The listing builds one solid part. Answer for the finished solid, in the listing's coordinates (mm). A direction names the side the tool comes from. Round coordinates to 2 decimals unless told otherwise and drop trailing zeros. Loops run counter-clockwise (first coordinate to the right, second up) from the corner with the lowest first, then second, coordinate; pieces in that order, holes last. Notation, with made-up numbers: M 22.5,27.25 L 70.5,27.25 A22 ccw 70.5,64.25 Z; hole C 75.25,81 d11. An arc over 180 degrees is marked long. Answer as a JSON object with one key per item and string values.
```python
from build123d import *

# Parameters (mm, degrees)
SKETCH1_R           = 48.26
BOSS_EXTRUDE1_DEPTH = 25.4
SKETCH2_R           = 8.382
CUT_EXTRUDE1_DEPTH  = 5.334
SKETCH12_R          = 6.731
CUT_EXTRUDE5_DEPTH  = 73.823177629
SKETCH15_R          = 6.731
BOSS_EXTRUDE2_DEPTH = 5.08
SKETCH16_R          = 1.5
CUT_EXTRUDE9_DEPTH  = 75.746809965
SKETCH14_R          = 6.858
CUT_EXTRUDE8_DEPTH  = 73.823177629


with BuildPart() as part:
    # Sketch1 → Boss-Extrude1 (new body)
    with BuildSketch(Plane.XY):
        Circle(SKETCH1_R)
    extrude(amount=BOSS_EXTRUDE1_DEPTH)

    # Sketch2 → Cut-Extrude1 (cut)
    with BuildSketch(Plane.XY.offset(25.4)):
        Circle(SKETCH2_R)
    cut_extrude1 = extrude(amount=-CUT_EXTRUDE1_DEPTH, mode=Mode.SUBTRACT)

    # Sketch12 → Cut-Extrude5 (cut, through all)
    with BuildSketch(Plane(origin=(0, 0, 0), x_dir=(-1, 0, 0), z_dir=(0, 0, -1))):
        with Locations((0, -15.24)):
            Circle(SKETCH12_R)
    extrude(amount=-CUT_EXTRUDE5_DEPTH, mode=Mode.SUBTRACT)

    # Sketch15 → Boss-Extrude2 (add)
    with BuildSketch(Plane.XY.offset(25.4)):
        with BuildLine():
            ThreePointArc((6.984961194, -4.633383333), (0, -8.382), (-6.984961194, -4.633383333))
            ThreePointArc((-6.984961194, -4.633383333), (0, -27.94), (6.984961194, -4.633383333))
        make_face()
        with Locations(Location((0, -15.24, 0), (0, 0, 180))):
            Circle(SKETCH15_R, mode=Mode.SUBTRACT)
    extrude(amount=BOSS_EXTRUDE2_DEPTH)

    # Sketch16 → Cut-Extrude9 (cut, through all)
    with BuildSketch(Plane.XY.offset(30.48)):
        with Locations((8.379661807, -10.402)):
            Circle(SKETCH16_R)
        with Locations((0, -24.916)):
            Circle(SKETCH16_R)
        with Locations((-8.379661807, -10.402)):
            Circle(SKETCH16_R)
    extrude(amount=-CUT_EXTRUDE9_DEPTH, mode=Mode.SUBTRACT)

    # Mirror1: Cut-Extrude1 across plane
    add(cut_extrude1.mirror(Plane.XY.offset(12.7)), mode=Mode.SUBTRACT)

    # Sketch14 → Cut-Extrude8 (cut, through all)
    with BuildSketch(Plane.XY.offset(25.4)):
        Circle(SKETCH14_R)
    extrude(amount=-CUT_EXTRUDE8_DEPTH, mode=Mode.SUBTRACT)


solid = part.part
```
Item 1: Flat-ended cylindrical pins translate along their axes: P1, Ø12, axis at y = 35.5, z = 6.5, coming from the -X side; P2, Ø2, axis at y = -17, z = 10.5, coming from the +X side; P3, Ø1.5, axis at x = 0.5, z = 8.5, coming from the -Y side; P4, Ø4, axis at x = -8.38, y = -10.4, coming from the +Z side. Find the tip coordinate at first contact, or state that the pin passes through.
Values follow:
{"P1": "x = -38.19", "P2": "x = 45.53", "P3": "y = -48.26", "P4": "z = 30.48"}
Item 2: Straight lines are drawn through the part: line 1 (Y direction, x = 0, z = 10); line 2 (Z direction, x = -22.5, y = -30.5); line 3 (X direction, y = -16, z = 7). For each, find the intervals that lie inside material, in ascending order.
Values follow:
{"line 1": "-48.26 to -26.42, -23.42 to -21.97, -8.51 to -6.86, 6.86 to 48.26", "line 2": "0 to 25.4", "line 3": "-45.53 to -6.69, 6.69 to 45.53"}
Item 3: Which of the six approach directions +Z, -Z, +X, -X, +Y, -Y give full straight-line access (tool end or side, diameter ignored) to faces 4 (the face through (-8.705, -11.866, 15.453)), 5 (the face through (1, -7, 20.066)), 6 (the face through (1, -7, 5.334))?
Values follow:
{"face 4": "+Z, -Z", "face 5": "+Z", "face 6": "-Z"}
Item 4: The part is cut by section A-A (x = 0). Give the vertices of the cut face in (y, z), then the cut area to 3 significant figures.
Values follow:
{"outline": "M -48.26,0 L -26.42,0 L -26.42,30.48 L -27.94,30.48 L -27.94,25.4 L -48.26,25.4 Z; M -23.42,0 L -21.97,0 L -21.97,30.48 L -23.42,30.48 Z; M -8.51,0 L -8.38,0 L -8.38,5.33 L -6.86,5.33 L -6.86,20.07 L -8.38,20.07 L -8.38,30.48 L -8.51,30.48 Z; M 6.86,5.33 L 8.38,5.33 L 8.38,0 L 48.26,0 L 48.26,25.4 L 8.38,25.4 L 8.38,20.07 L 6.86,20.07 Z", "area": "1,670 mm^2"}
Item 5: Determine the mould class of faces 1 (the face through (-1.487, -6.695, 12.803)), 2 (the face through (-0.455, -27.932, 27.904)), 3 (the face through (-6, -19, 30.48)) for opening direction Y: released by +Y, released by -Y, zero draft, split by the parting line, or undercut.
Values follow:
{"face 1": "undercut", "face 2": "split by the parting line", "face 3": "zero draft"}
Item 6: The part is cut by section C-C (y = -18.5). Give the vertices of the cut face in (x, z), then the cut area to 3 significant figures.
Values follow:
{"outline": "M -44.57,0 L -5.89,0 L -5.89,30.48 L -12.27,30.48 L -12.27,25.4 L -44.57,25.4 Z; M 5.89,0 L 44.57,0 L 44.57,25.4 L 12.27,25.4 L 12.27,30.48 L 5.89,30.48 Z", "area": "2,030 mm^2"}
Item 7: The part is cut by section B-B (y = 0). Give the vertices of the cut face in (x, z).
Values follow:
{"outline": "M -48.26,0 L -8.38,0 L -8.38,5.33 L -6.86,5.33 L -6.86,20.07 L -8.38,20.07 L -8.38,25.4 L -48.26,25.4 Z; M 6.86,5.33 L 8.38,5.33 L 8.38,0 L 48.26,0 L 48.26,25.4 L 8.38,25.4 L 8.38,20.07 L 6.86,20.07 Z"}
Item 8: The part is cut by section D-D (z = 3.5). Give the vertices of the cut face in (x, y), then the cut area to 3 significant figures.
Values follow:
{"outline": "C 0,0 d96.52; hole C -8.38,-10.4 d3; hole C 0,0 d16.76; hole C 0,-15.24 d13.46; hole C 0,-24.92 d3; hole C 8.38,-10.4 d3", "area": "6,930 mm^2"}
